Verification items for the finished model (mm, model axes). A direction names the side the tool comes from. Give positions to 0.01 mm unless a question says otherwise; leave off trailing zeros. Loops run counter-clockwise (first coordinate to the right, second up) from the corner with the lowest first, then second, coordinate; pieces in that order, holes last. Notation, with made-up numbers: (54, 49.5) - (66, 49.5) arc R21 ccw to (66, 57.5) - close; hole circle Ø6 at (-25.75, 42.25). An arc over 180 degrees is marked (long way). Answer in a Markdown table with one row per item.
```python
from build123d import *

# Parameters (mm, degrees)
BOSS_EXTRUDE1_DEPTH = 42
CUT_EXTRUDE2_DEPTH  = 58.425262324
FILLET1_R           = 1


with BuildPart() as part:
    # Sketch1 → Boss-Extrude1 (new body)
    with BuildSketch(Plane.XY):
        with BuildLine():
            Line((0, 0), (3, 8.626746371))
            Line((3, 8.626746371), (6, 8.626746371))
            Line((6, 8.626746371), (6, 6.626746371))
            Line((6, 6.626746371), (5, 6.626746371))
            Line((5, 6.626746371), (5, 3.926746371))
            Line((5, 3.926746371), (33.2, 3.926746371))
            Line((33.2, 3.926746371), (33.2, 6.626746371))
            Line((33.2, 6.626746371), (32.2, 6.626746371))
            Line((32.2, 6.626746371), (32.2, 8.626746371))
            Line((32.2, 8.626746371), (35.2, 8.626746371))
            Line((35.2, 8.626746371), (38.2, 0))
            ThreePointArc((38.2, 0), (19.1, 2.426746371), (0, 0))
        make_face()
    extrude(amount=BOSS_EXTRUDE1_DEPTH)

    # Sketch5 → Cut-Extrude2 (cut, through all)
    with BuildSketch(Plane(origin=(0, 0, 0), x_dir=(0, 0, -1), z_dir=(1, 0, 0))):
        Polygon((-42, 0), (-42, 8.626746371), (-37, 8.626746371), align=None)
        Polygon((0, 0), (0, 8.626746371), (-2.959406662, 8.626746371), align=None)
    extrude(amount=CUT_EXTRUDE2_DEPTH, mode=Mode.SUBTRACT)

    # Fillet1
    fillet1_edges = [part.edges().sort_by_distance(p)[0] for p in [
        (32.2, 7.626746371, 2.616356509),
        (33.2, 5.276746371, 1.81018865),
        (36.7, 4.313373185, 1.479703331),
        (33.7, 8.626746371, 2.959406662),
        (3, 8.626746371, 19.979703331),
        (4.5, 8.626746371, 2.959406662),
        (19.1, 3.926746371, 1.347070943),
        (5, 5.276746371, 1.81018865),
        (6, 7.626746371, 2.616356509),
        (36.7, 4.313373185, 39.5),
        (1.5, 4.313373185, 39.5),
        (35.2, 8.626746371, 19.979703331),
        (6, 8.626746371, 19.979703331),
        (4.5, 8.626746371, 37),
        (6, 7.626746371, 37.57959279),
        (5, 5.276746371, 38.941635847),
        (32.2, 8.626746371, 19.979703331),
        (33.7, 8.626746371, 37),
        (32.2, 7.626746371, 37.57959279),
        (33.2, 5.276746371, 38.941635847),
        (19.1, 3.926746371, 39.724086114),
    ]]
    fillet(fillet1_edges, radius=FILLET1_R - 0.0001)  # a hair under: the kernel refuses the full size


solid = part.part
```
Q1. Sectioned sample at C-C (x = 13.5). Record the cut outline in (y, z).
Completed:
| item | result |
|---|---|
| outline | (2.22, 0.76) - (3.25, 1.12) arc R1 ccw to (3.93, 2.06) - (3.93, 39.15) arc R1 ccw to (3.43, 40.01) - (2.22, 40.71) - close |
Q2. Thickness scan on line 1 (X direction, y = 6, z = 8.5); line 2 (Y direction, x = 24, z = 38); line 3 (X direction, y = 4.25, z = 29). Record the ranges inside material, lowest first.
Completed:
| item | result |
|---|---|
| line 1 | 2.09 to 5, 33.2 to 36.11 |
| line 2 | 2.27 to 3.93 |
| line 3 | 1.48 to 5, 33.2 to 36.72 |
Q3. Go/stop test with flat-tipped pins: P1, Ø5, axis at y = 4, z = 20, coming from the -X side; P2, Ø2, axis at y = 2, z = 6.5, coming from the +X side; P3, Ø0.8, axis at y = 7, z = 17.5, coming from the -X side. Record where each tip stops, or that it passes through.
Completed:
| item | result |
|---|---|
| P1 | x = 0.52 |
| P2 | x = 37.85 |
| P3 | x = 2.3 |
Q4. Sectioned sample at B-B (x = 19). Record the cut outline in (y, z).
Completed:
| item | result |
|---|---|
| outline | (2.43, 0.83) - (3.25, 1.12) arc R1 ccw to (3.93, 2.06) - (3.93, 39.15) arc R1 ccw to (3.43, 40.01) - (2.43, 40.59) - close |
Q5. Sectioned sample at A-A (z = 11). Record the cut outline in (x, y).
Completed:
| item | result |
|---|---|
| outline | (0, 0) arc R76.38 cw to (38.2, 0) - (35.43, 7.96) arc R1 ccw to (34.49, 8.63) - (33.2, 8.63) arc R1 ccw to (32.2, 7.63) - (32.2, 6.63) - (33.2, 6.63) - (33.2, 3.93) - (5, 3.93) - (5, 6.63) - (6, 6.63) - (6, 7.63) arc R1 ccw to (5, 8.63) - (3.71, 8.63) arc R1 ccw to (2.77, 7.96) - close |
Q6. Draft check along X on faces 4 (the face through (36.49, 4.18, 39.31)), 5 (the face through (1.656, 4.061, 39.365)), 6 (the face through (32.501, 7.224, 37.483)). Enter one of: +X half, -X half, draft (parallel to the pull), parting line (faces both ways), or undercut.
Completed:
| item | result |
|---|---|
| face 4 | +X half |
| face 5 | -X half |
| face 6 | undercut |
Q7. Tool access check on faces 1 (the face through (5.7, 7.25, 37.47)), 2 (the face through (4.7, 5.03, 2.03)), 3 (the face through (4.7, 5.16, 38.68)). Record the directions out of +Z, -Z, +X, -X, +Y, -Y that give a thin tool (end or side, any length) a straight path to the whole face; none if there is none.
Completed:
| item | result |
|---|---|
| face 1 | +Z, +Y |
| face 2 | -Z |
| face 3 | +Z |
